The listing builds one solid part. Answer for the finished solid, in the listing's coordinates (mm). A direction names the side the tool comes from. Coordinates: 2 decimals unless noted, no trailing zeros. Order: outer loops, then holes, each group sorted by start corner. A loop starts at its lowest first (then second) coordinate and runs counter-clockwise, first axis right, second up. Notation, with made-up numbers: (6, 2.25) -> (39, 2.25) arc R28 cw to (39, 21.25) -> close; hole circle Ø3 at (78, 25.25). An arc over 180 degrees is marked (long way). Put each result on its own line as item: value. Start each with the question number.
```python
from build123d import *

# Parameters (mm, degrees)
F0_R          = 3
F0_R_2        = 2.5
F1_DEPTH      = 180
F2_R          = 2
F3_R          = 7
F6_DEPTH      = 30
F6_DEPTH_BACK = 30


# Not quite as in the source:
# - a feature names something its author has since deleted; it is built from what else it names


with BuildPart() as f1:
    # F0 (on Top) → F1 (new body)
    with BuildSketch(Plane.XY):
        with BuildLine():
            Line((18.15, -30), (30, -30))
            Line((30, -30), (30, -18.15))
            Line((30, -18.15), (27.5, -18.15))
            Line((27.5, -18.15), (27.5, -20.15))
            Line((27.5, -20.15), (21.5477069044, -20.15))
            ThreePointArc((21.5477069044, -20.15), (19.5, -15), (21.5477069044, -9.85))
            Line((21.5477069044, -9.85), (27.5, -9.85))
            Line((27.5, -9.85), (27.5, -11.85))
            Line((27.5, -11.85), (30, -11.85))
            Line((30, -11.85), (30, 11.85))
            Line((30, 11.85), (27.5, 11.85))
            Line((27.5, 11.85), (27.5, 9.85))
            Line((27.5, 9.85), (21.5477069044, 9.85))
            ThreePointArc((21.5477069044, 9.85), (19.5, 15), (21.5477069044, 20.15))
            Line((21.5477069044, 20.15), (27.5, 20.15))
            Line((27.5, 20.15), (27.5, 18.15))
            Line((27.5, 18.15), (30, 18.15))
            Line((30, 18.15), (30, 30))
            Line((30, 30), (18.15, 30))
            Line((18.15, 30), (18.15, 27.5))
            Line((18.15, 27.5), (20.15, 27.5))
            Line((20.15, 27.5), (20.15, 21.5477069044))
            ThreePointArc((20.15, 21.5477069044), (15, 19.5), (9.85, 21.5477069044))
            Line((9.85, 21.5477069044), (9.85, 27.5))
            Line((9.85, 27.5), (11.85, 27.5))
            Line((11.85, 27.5), (11.85, 30))
            Line((11.85, 30), (-11.85, 30))
            Line((-11.85, 30), (-11.85, 27.5))
            Line((-11.85, 27.5), (-9.85, 27.5))
            Line((-9.85, 27.5), (-9.85, 21.5477069044))
            ThreePointArc((-9.85, 21.5477069044), (-15, 19.5), (-20.15, 21.5477069044))
            Line((-20.15, 21.5477069044), (-20.15, 27.5))
            Line((-20.15, 27.5), (-18.15, 27.5))
            Line((-18.15, 27.5), (-18.15, 30))
            Line((-18.15, 30), (-30, 30))
            Line((-30, 30), (-30, 18.15))
            Line((-30, 18.15), (-27.5, 18.15))
            Line((-27.5, 18.15), (-27.5, 20.15))
            Line((-27.5, 20.15), (-21.5477069044, 20.15))
            ThreePointArc((-21.5477069044, 20.15), (-19.5, 15), (-21.5477069044, 9.85))
            Line((-21.5477069044, 9.85), (-27.5, 9.85))
            Line((-27.5, 9.85), (-27.5, 11.85))
            Line((-27.5, 11.85), (-30, 11.85))
            Line((-30, 11.85), (-30, -11.85))
            Line((-30, -11.85), (-27.5, -11.85))
            Line((-27.5, -11.85), (-27.5, -9.85))
            Line((-27.5, -9.85), (-21.5477069044, -9.85))
            ThreePointArc((-21.5477069044, -9.85), (-19.5, -15), (-21.5477069044, -20.15))
            Line((-21.5477069044, -20.15), (-27.5, -20.15))
            Line((-27.5, -20.15), (-27.5, -18.15))
            Line((-27.5, -18.15), (-30, -18.15))
            Line((-30, -18.15), (-30, -30))
            Line((-30, -30), (-18.15, -30))
            Line((-18.15, -30), (-18.15, -27.5))
            Line((-18.15, -27.5), (-20.15, -27.5))
            Line((-20.15, -27.5), (-20.15, -21.5477069044))
            ThreePointArc((-20.15, -21.5477069044), (-15, -19.5), (-9.85, -21.5477069044))
            Line((-9.85, -21.5477069044), (-9.85, -27.5))
            Line((-9.85, -27.5), (-11.85, -27.5))
            Line((-11.85, -27.5), (-11.85, -30))
            Line((-11.85, -30), (11.85, -30))
            Line((11.85, -30), (11.85, -27.5))
            Line((11.85, -27.5), (9.85, -27.5))
            Line((9.85, -27.5), (9.85, -21.5477069044))
            ThreePointArc((9.85, -21.5477069044), (15, -19.5), (20.15, -21.5477069044))
            Line((20.15, -21.5477069044), (20.15, -27.5))
            Line((20.15, -27.5), (18.15, -27.5))
            Line((18.15, -27.5), (18.15, -30))
        make_face()
        with Locations((-25, -25)):
            Circle(F0_R, mode=Mode.SUBTRACT)
        with Locations((-15, -15)):
            Circle(F0_R_2, mode=Mode.SUBTRACT)
        with Locations((25, -25)):
            Circle(F0_R, mode=Mode.SUBTRACT)
        with Locations((15, -15)):
            Circle(F0_R_2, mode=Mode.SUBTRACT)
        with Locations((-25, 25)):
            Circle(F0_R, mode=Mode.SUBTRACT)
        with Locations((-15, 15)):
            Circle(F0_R_2, mode=Mode.SUBTRACT)
        Polygon((-7, 22), (-7, 27.5), (0, 27.5), (7, 27.5), (7, 22), (10, 16), (10, 10), (16, 10), (22, 7), (27.5, 7), (27.5, 0), (27.5, -7), (22, -7), (16, -10), (10, -10), (10, -16), (7, -22), (7, -27.5), (0, -27.5), (-7, -27.5), (-7, -22), (-10, -16), (-10, -10), (-16, -10), (-22, -7), (-27.5, -7), (-27.5, 0), (-27.5, 7), (-22, 7), (-16, 10), (-10, 10), (-10, 16), align=None, mode=Mode.SUBTRACT)
        with Locations((15, 15)):
            Circle(F0_R_2, mode=Mode.SUBTRACT)
        with Locations((25, 25)):
            Circle(F0_R, mode=Mode.SUBTRACT)
    extrude(amount=F1_DEPTH)

    # F2
    f2_edges = [f1.edges().sort_by_distance(p)[0] for p in [
        (-7, 27.5, 90),
        (7, 27.5, 90),
    ]]
    fillet(f2_edges, radius=F2_R)

    # F3
    f3_edges = [f1.edges().sort_by_distance(p)[0] for p in [
        (-10, 16, 90),
        (10, 16, 90),
    ]]
    fillet(f3_edges, radius=F3_R)

    # F5 (on Front) → F6 (cut, two sides)
    with BuildSketch(Plane.XZ) as f6_sk:
        Polygon((79.680713533, 21.8168503847), (-30, 0), (-17.5886362159, -62.3961393031), (92.0920773171, -40.5792889183), align=None)
        Polygon((97.6667223127, 202.7474358776), (-20.7884412878, 226.3096328978), (-30, 180), (88.4551636005, 156.4378029799), align=None)
    extrude(amount=F6_DEPTH, mode=Mode.SUBTRACT)
    extrude(f6_sk.sketch, amount=-F6_DEPTH_BACK, mode=Mode.SUBTRACT)


solid = f1.part
```
(1) The part is cut by section A-A on x = -2.5. Determine the outline of the cut face in (y, z), plus the area to 3 significant figures.
(2) The part is cut by section B-B on x = -25. Determine the outline of the cut face in (y, z), plus the area to 3 significant figures.
(3) This flat-tipped pin is pushed along its axis until it touches: P1, Ø3, axis at x = 14.5, z = 78.5, coming from the -Y side. Where does it stop, or does it pass through?
(4) The part is cut by section C-C on z = 73. Count the separate pieces of the cut face and the enclosed holes in it, plus the area to 3 significant figures.
(5) Find the intervals of material crossed by L1, parallel to X at y = 15, z = 127.5; L2, parallel to Y at x = 15, z = 76; L3, parallel to X at y = 25, z = 91.5, in increasing order.
(6) For a pull along X with two mould halves and no side action, classify faces 1 (the flat face through (-24, -30, 89)), 2 (the flat face through (-20.15, -25, 89)), 3 (the flat face through (-30, -24, 89)) as released by +X, released by -X, zero draft, split by the parting line, or undercut.
(7) A tool of negligible diameter and unlimited length cuts with its end or side. For faces 4 (the flat face through (24, -30, 89)), 5 (the flat face through (-10, -13, 89)), from which of +Z, -Z, +X, -X, +Y, -Y can it reach the whole face along a straight path? Write none if from no direction.
Worked out:
1. outline: (-30, 5.47) -> (-27.5, 5.47) -> (-27.5, 174.53) -> (-30, 174.53) -> close; (27.5, 5.47) -> (30, 5.47) -> (30, 174.53) -> (27.5, 174.53) -> close
1. area: 845 mm2
2. outline: (-30, 0.99) -> (-28, 0.99) -> (-28, 179.01) -> (-30, 179.01) -> close; (-22, 0.99) -> (-20.15, 0.99) -> (-20.15, 179.01) -> (-22, 179.01) -> close; (-9.85, 0.99) -> (-7, 0.99) -> (-7, 179.01) -> (-9.85, 179.01) -> close; (7, 0.99) -> (9.85, 0.99) -> (9.85, 179.01) -> (7, 179.01) -> close; (20.15, 0.99) -> (22, 0.99) -> (22, 179.01) -> (20.15, 179.01) -> close; (28, 0.99) -> (30, 0.99) -> (30, 179.01) -> (28, 179.01) -> close
2. area: 2,390 mm2
3. P1: y = -19.77
4. separate pieces: 1
4. enclosed holes: 9
4. area: 1,080 mm2
5. L1: -19.5 to -17.5, -12.5 to -9.97, 9.97 to 12.5, 17.5 to 19.5
5. L2: -19.5 to -17.5, -12.5 to -10, 10 to 12.5, 17.5 to 19.5
5. L3: -30 to -28, -22 to -20.15, -9.85 to -7, 7 to 9.85, 20.15 to 22, 28 to 30
6. face 1: zero draft
6. face 2: undercut
6. face 3: released by -X
7. face 4: +Z, -Z, +X, -X, -Y
7. face 5: +Z, -Z
